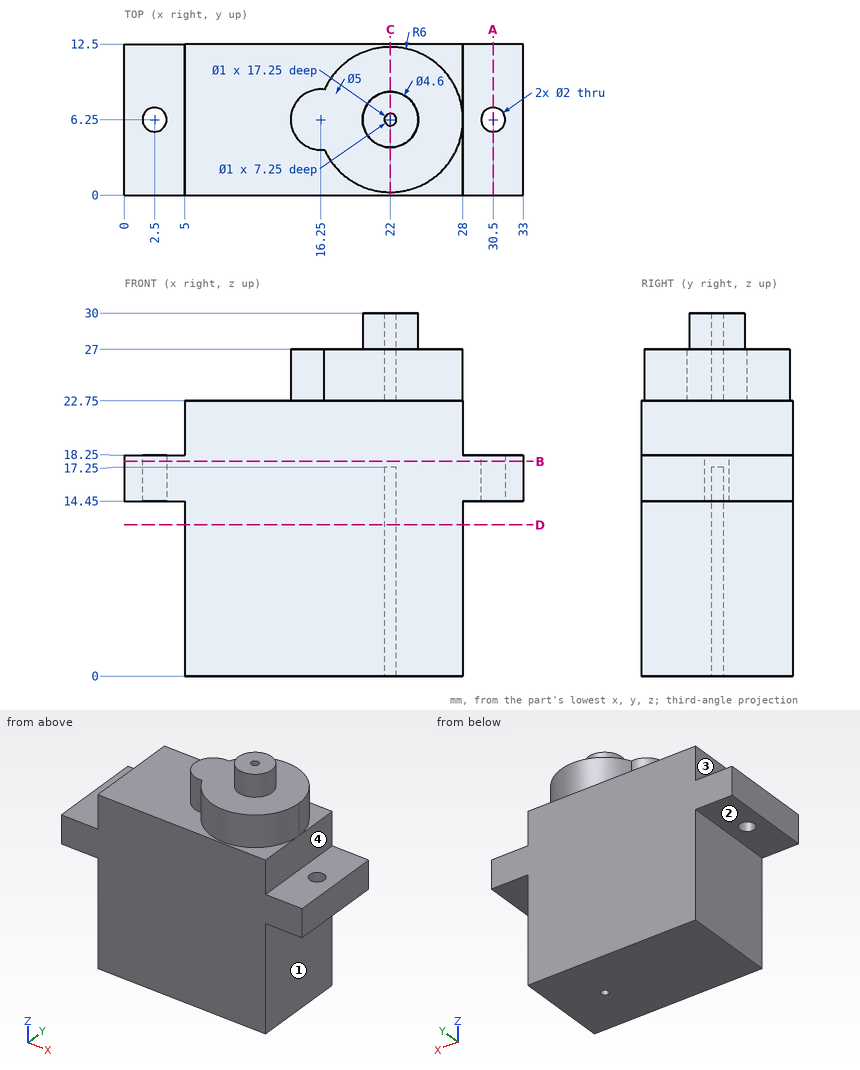
Can you work these out from the drawing? Everything is in mm from the part's minimum corner. A direction names the side the tool comes from. Round coordinates to 2 decimals unless told otherwise and drop trailing zeros. Loops run counter-clockwise (first coordinate to the right, second up) from the corner with the lowest first, then second, coordinate; pieces in that order, holes last. Notation, with made-up numbers: (-32.5, -36.75) -> (10.5, -36.75) arc R36 ccw to (10.5, 2.25) -> close; hole circle Ø8 at (-10.75, 27.5). An arc over 180 degrees is marked (long way). Put each result on its own line as item: value.
Q1. I want a section at B-B on z = 17.75. Write out the boundary of the cut face in (x, y).
Checks:
outline: (0, 0) -> (33, 0) -> (33, 12.5) -> (0, 12.5) -> close; hole circle Ø2 at (2.5, 6.25); hole circle Ø2 at (30.5, 6.25)
Q2. I want a section at C-C on x = 22. Write out the boundary of the cut face in (y, z).
Checks:
outline: (0, 0) -> (5.75, 0) -> (5.75, 17.25) -> (6.75, 17.25) -> (6.75, 0) -> (12.5, 0) -> (12.5, 22.75) -> (12.25, 22.75) -> (12.25, 27) -> (8.55, 27) -> (8.55, 30) -> (6.75, 30) -> (6.75, 22.75) -> (5.75, 22.75) -> (5.75, 30) -> (3.95, 30) -> (3.95, 27) -> (0.25, 27) -> (0.25, 22.75) -> (0, 22.75) -> close
Q3. For pin 1 Ø2.5 at (x, y) = (30, 6.5) entering from -Z; pin 2 Ø1 at (x, z) = (12, 8.5) entering from -Y; pin 3 Ø1.5 at (x, y) = (30.5, 5) entering from +Z; pin 4 Ø3 at (x, y) = (13.5, 11) entering from +Z, each with a flat end and sliding along its axis, tell me the tip position at first contact or that it passes through.
Checks:
pin 1: z = 14.45
pin 2: y = 0
pin 3: z = 18.25
pin 4: z = 22.75
Q4. I want a section at A-A on x = 30.5. Write out the boundary of the cut face in (y, z), and give its area (3 significant figures).
Checks:
outline: (0, 14.45) -> (5.25, 14.45) -> (5.25, 18.25) -> (0, 18.25) -> close; (7.25, 14.45) -> (12.5, 14.45) -> (12.5, 18.25) -> (7.25, 18.25) -> close
area: 39.9 mm2
Q5. Please list where these lines run through material, in increasing order: line 1 (Y direction, x = 22, z = 5.75); line 2 (Y direction, x = 2.5, z = 16.7); line 3 (X direction, y = 3, z = 4.75). Write a range as from..to.
Checks:
line 1: 0..5.75, 6.75..12.5
line 2: 0..5.25, 7.25..12.5
line 3: 5..28
Q6. I want a section at D-D on z = 12.5. Write out the boundary of the cut face in (x, y).
Checks:
outline: (5, 0) -> (28, 0) -> (28, 12.5) -> (5, 12.5) -> close; hole circle Ø1 at (22, 6.25)
Q7. Which directions (+Z, -Z, +X, -X, +Y, -Y) give clear straight access to the entire face, cutting with the end or side of a thin tool? Please do the marked faces 1, 2, 3 and 4.
Checks:
face 1: -Z, +X, +Y, -Y
face 2: -Z, -X, +Y, -Y
face 3: +Z, -X, +Y, -Y
face 4: +Z, +X, +Y, -Y
